```python
from build123d import *

# Parameters (mm, degrees)
SKETCH2_R           = 31.115
BOSS_EXTRUDE1_DEPTH = 12.7
SKETCH3_R           = 2.0828
CUT_EXTRUDE3_DEPTH  = 12.7
SKETCH4_R           = 22.225
CUT_EXTRUDE2_DEPTH  = 6.35
CUT_EXTRUDE4_REACH  = 49.95
SKETCH8_R           = 0.79375
CIRPATTERN1_COUNT   = 3


with BuildPart() as part:
    # Sketch2 → Boss-Extrude1 (new body)
    with BuildSketch(Plane(origin=(0, 0, -1.71308935), x_dir=(-1, 0, 0), z_dir=(0, 0, -1))):
        Circle(SKETCH2_R)
    extrude(amount=BOSS_EXTRUDE1_DEPTH)

    # Sketch3 → Cut-Extrude3 (cut)
    with BuildSketch(Plane(origin=(0, 0, -14.41308935), x_dir=(-1, 0, 0), z_dir=(0, 0, -1))):
        with Locations((0, 26.67)):
            Circle(SKETCH3_R)
        with Locations((18.858537854, 18.858537854)):
            Circle(SKETCH3_R)
        with Locations((26.67, 0)):
            Circle(SKETCH3_R)
        with Locations((18.858537854, -18.858537854)):
            Circle(SKETCH3_R)
        with Locations((0, -26.67)):
            Circle(SKETCH3_R)
        with Locations((-18.858537854, -18.858537854)):
            Circle(SKETCH3_R)
        with Locations((-26.67, 0)):
            Circle(SKETCH3_R)
        with Locations((-18.858537854, 18.858537854)):
            Circle(SKETCH3_R)
    extrude(amount=-CUT_EXTRUDE3_DEPTH, mode=Mode.SUBTRACT)

    # Sketch4 → Cut-Extrude2 (cut)
    with BuildSketch(Plane.XY.offset(-1.71308935)):
        Circle(SKETCH4_R)
    extrude(amount=-CUT_EXTRUDE2_DEPTH, mode=Mode.SUBTRACT)

    # Sketch6 → Cut-Revolve2 (revolve, cut)
    with BuildSketch(Plane(origin=(0, 0, 0), x_dir=(0, 0, -1), z_dir=(1, 0, 0)), mode=Mode.PRIVATE) as cut_revolve2_sk:
        Polygon((9.96808935, 0), (9.96808935, 6.35), (12.50808935, 6.35), (12.50808935, 2.0828), (14.41308935, 2.0828), (14.41308935, 0), align=None)
    revolve(cut_revolve2_sk.sketch.rotate(Axis((0, 0, 69.036833432), (0, 0, -1)), 90), axis=Axis((0, 0, 69.036833432), (0, 0, -1)), mode=Mode.SUBTRACT)

    # Cut-Extrude4: up to this plane
    cut_extrude4_end = Plane(origin=(0, 0, -9.96808935), z_dir=(0, 0, -1))
    # Sketch8 → Cut-Extrude4 (cut, up to the surface)
    with BuildSketch(Plane(origin=(0, 0, 4.63691065), x_dir=(1, 0, 0), z_dir=(0, -0.21242964433104367, 0.9771763639228009)), mode=Mode.PRIVATE) as cut_extrude4_sk1:
        with Locations(Location((0, 0, 0), (0, 0, 270))):
            Circle(SKETCH8_R)
    cut_extrude4_tool1 = split(extrude(cut_extrude4_sk1.sketch, amount=-CUT_EXTRUDE4_REACH, mode=Mode.PRIVATE), bisect_by=cut_extrude4_end, keep=Keep.BOTH, mode=Mode.PRIVATE)
    cut_extrude4 = cut_extrude4_tool1.solids().sort_by_distance((0, 0, 4.636911))[0]
    add(cut_extrude4, mode=Mode.SUBTRACT)

    # CirPattern1: Cut-Extrude4 ×3 about axis
    cirpattern1_axis = Axis((0, 0, -1.71308935), (0, 0, 1))
    for i in range(1, CIRPATTERN1_COUNT):
        add(cut_extrude4.rotate(cirpattern1_axis, i * 360 / CIRPATTERN1_COUNT), mode=Mode.SUBTRACT)


solid = part.part
```
CAD build for the part. Positions are in the model's coordinates, mm. A direction names the side the tool comes from. Give positions to 0.01 mm unless a question says otherwise; leave off trailing zeros. Loops run counter-clockwise (first coordinate to the right, second up) from the corner with the lowest first, then second, coordinate; pieces in that order, holes last. Notation, with made-up numbers: (-3, -24.5) - (2, -24.5) arc R15 ccw to (2, 0.5) - close; hole circle Ø7 at (48, 34.5). An arc over 180 degrees is marked (long way). Put each result on its own line as item: value.
Q1. Slice it at B-B (z = -7). Give the number of separate pieces and of enclosed holes in the cut face, plus the area to 3 significant figures.
Filled in:
separate pieces: 1
enclosed holes: 9
area: 1,380 mm²
Q2. Probe line 1 along Y through (x, z) = (0, -11.3) (3 decimals); line 2 along Z through (x, y) = (0, 5); line 3 along X through (y, z) = (-19, -5.5). List the from-to ranges inside material, lowest first.
Filled in:
line 1: y = -31.115 to -28.753, -24.587 to -6.35, 6.35 to 24.587, 28.753 to 31.115
line 2: z = -14.41 to -12.51, -9.97 to -8.06
line 3: x = -24.64 to -20.94, -16.78 to -11.53, 11.53 to 16.78, 20.94 to 24.64
Q3. Slice it at C-C (y = 26.67). Give the cut face in (x, z).
Filled in:
outline: (-16.03, -14.41) - (-2.08, -14.41) - (-2.08, -1.71) - (-16.03, -1.71) - close; (2.08, -14.41) - (16.03, -14.41) - (16.03, -1.71) - (2.08, -1.71) - close
Q4. Flat gauge pins, fed straight in: pin 1 (14 mm diameter, centred on x = -0.5, y = -2, fed in from +Z); pin 2 (5 mm diameter, centred on y = 23.5, z = -12, fed in from -X); pin 3 (1.5 mm diameter, centred on x = 18.5, z = -6.5, fed in from +Y); pin 4 (2.5 mm diameter, centred on x = 18.86, y = -18.86, fed in from -Z). Where does each tip first touch, or does it go through?
Filled in:
pin 1: stops at z = -8.06
pin 2: stops at x = -22.96
pin 3: stops at y = 25.56
pin 4: passes through
Q5. Slice it at D-D (x = -18). Give the cut face in (y, z), plus the area to 3 significant figures.
Filled in:
outline: (-25.38, -14.41) - (-20.76, -14.41) - (-20.76, -1.71) - (-25.38, -1.71) - close; (-16.96, -14.41) - (16.96, -14.41) - (16.96, -1.71) - (13.04, -1.71) - (13.04, -8.06) - (-13.04, -8.06) - (-13.04, -1.71) - (-16.96, -1.71) - close; (20.76, -14.41) - (25.38, -14.41) - (25.38, -1.71) - (20.76, -1.71) - close
area: 383 mm²
Q6. Slice it at A-A (x = 0). Give the cut face in (y, z) (3 decimals).
Filled in:
outline: (-31.115, -14.413) - (-28.753, -14.413) - (-28.753, -1.713) - (-31.115, -1.713) - close; (-24.587, -14.413) - (-2.083, -14.413) - (-2.083, -12.508) - (-6.35, -12.508) - (-6.35, -9.968) - (2.363, -9.968) - (1.949, -8.063) - (-22.225, -8.063) - (-22.225, -1.713) - (-24.587, -1.713) - close; (2.083, -14.413) - (24.587, -14.413) - (24.587, -1.713) - (22.225, -1.713) - (22.225, -8.063) - (3.573, -8.063) - (3.987, -9.968) - (6.35, -9.968) - (6.35, -12.508) - (2.083, -12.508) - close; (28.753, -14.413) - (31.115, -14.413) - (31.115, -1.713) - (28.753, -1.713) - close
Q7. Mould opens along X. For faces 1 (the face through (-9, -21, -1.713)), 2 (the face through (19.31, 16.825, -8.152)), 3 (the face through (6.745, -30.375, -7.974)) say: pulls with the +X half, pulls with the -X half, needs draft (parallel to the pull), parting line crosses it, or undercut.
Filled in:
face 1: needs draft
face 2: undercut
face 3: parting line crosses it
Q8. Tool access for faces 4 (the face through (1.987, -0.626, -13.474)), 5 (the face through (21.199, 6.676, -4.844)), 6 (the face through (-28.594, -0.798, -8.152)), 7 (the face through (0, -6, -14.413)), 8 (the face through (0, 0, -9.968)): list every direction of +Z, -Z, +X, -X, +Y, -Y with a clear straight run to the whole face (end or side of a thin tool).
Filled in:
face 4: -Z
face 5: +Z
face 6: +Z, -Z
face 7: -Z, +X, -X, +Y, -Y
face 8: none
